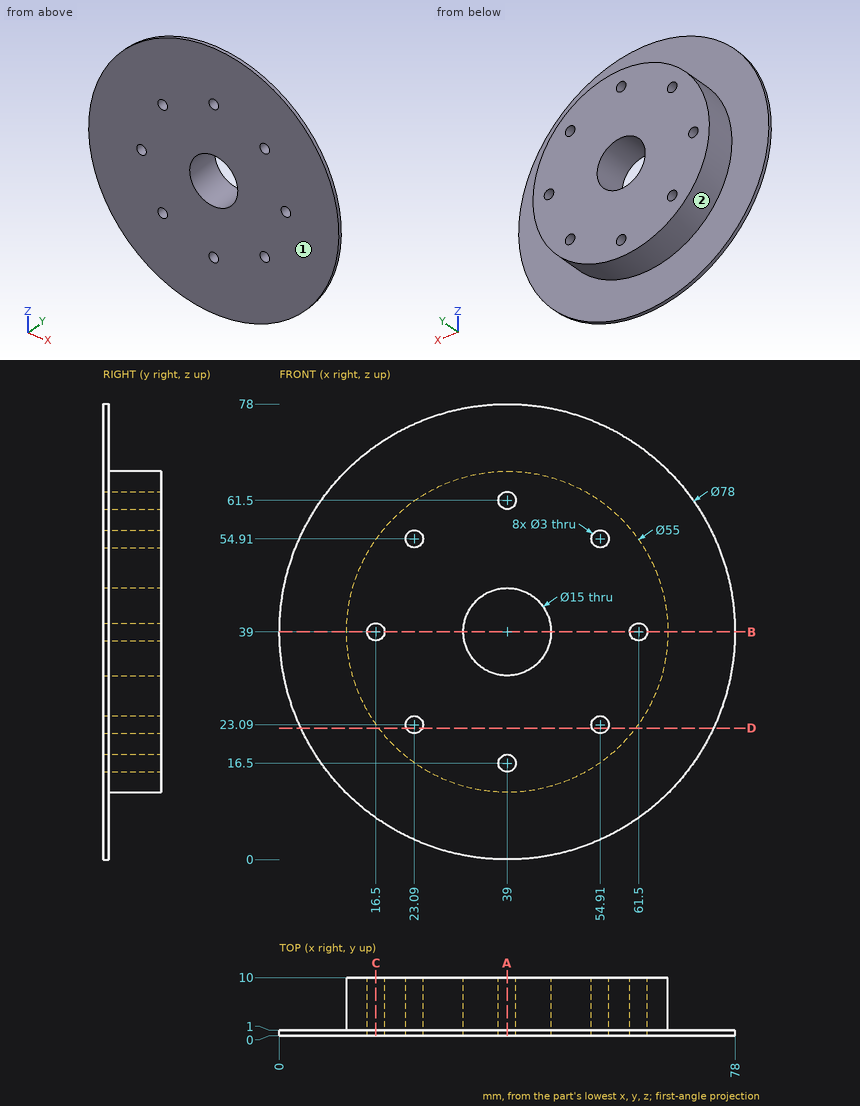
The figure shows three views and two pictorial views of one solid part (mm, origin at its lowest corner). Answer the questions. A direction names the side the tool comes from. Give positions to 0.01 mm unless a question says otherwise; leave off trailing zeros. Write each loop counter-clockwise with the first axis right and the second up, starting at its lowest first coordinate (ties: lowest second). Pieces come first, ordered by that corner, then holes. Notation, with made-up numbers: M 26.5,-11 L 71.5,-11 A24 cw 71.5,25 Z; hole C 8.5,45.25 d11. An arc over 180 degrees is marked long. One line per item, written item: value. Start each with the question number.
(1) Find section D-D (z = 22.5). Determine the outline of the cut face in (x, y).
(2) Find section C-C (x = 16.5). Determine the outline of the cut face in (y, z) (1 decimal), plus the area to 3 significant figures.
(3) Flat-ended cylindrical pins translate along their axes: pin 1 Ø3 at (y, z) = (6.5, 34.5) entering from +X; pin 2 Ø5 at (y, z) = (4, 62) entering from +X; pin 3 Ø5 at (y, z) = (4.5, 27) entering from -X. Find the tip coordinate at first contact, or state that the pin passes through.
(4) Find section B-B (z = 39). Determine the outline of the cut face in (x, y).
(5) Find section A-A (x = 39). Determine the outline of the cut face in (y, z).
(6) A tool of negligible diameter and unlimited length cuts with its end or side. For the marked faces 1 and 2, from which of +Z, -Z, +X, -X, +Y, -Y can it reach the whole face along a straight path? Write none if from no direction.
(7) Find the intervals of material crossed by line 1 (X direction, y = 2.5, z = 39); line 2 (X direction, y = 4.25, z = 54); line 3 (Z direction, x = 38.5, y = 1.75), in increasing order.
Results below:
1. outline: M 3.66,0 L 21.71,0 L 21.71,10 L 17,10 L 17,1 L 3.66,1 Z; M 24.47,0 L 53.53,0 L 53.53,10 L 24.47,10 Z; M 56.29,0 L 74.34,0 L 74.34,1 L 61,1 L 61,10 L 56.29,10 Z
2. outline: M 0,7.1 L 1,7.1 L 1,23.2 L 10,23.2 L 10,37.5 L 0,37.5 Z; M 0,40.5 L 10,40.5 L 10,54.8 L 1,54.8 L 1,70.9 L 0,70.9 Z
2. area: 318 mm^2
3. pin 1: stops at x = 66.34
3. pin 2: stops at x = 57.33
3. pin 3: stops at x = 13.19
4. outline: M 0,0 L 15,0 L 15,10 L 11.5,10 L 11.5,1 L 0,1 Z; M 18,0 L 31.5,0 L 31.5,10 L 18,10 Z; M 46.5,0 L 60,0 L 60,10 L 46.5,10 Z; M 63,0 L 78,0 L 78,1 L 66.5,1 L 66.5,10 L 63,10 Z
5. outline: M 0,0 L 1,0 L 1,11.5 L 10,11.5 L 10,15 L 0,15 Z; M 0,18 L 10,18 L 10,31.5 L 0,31.5 Z; M 0,46.5 L 10,46.5 L 10,60 L 0,60 Z; M 0,63 L 10,63 L 10,66.5 L 1,66.5 L 1,78 L 0,78 Z
6. face 1: +Z, -Z, +X, -X, -Y
6. face 2: +Y
7. line 1: x = 11.5 to 15, 18 to 31.5, 46.5 to 60, 63 to 66.5
7. line 2: x = 15.95 to 21.9, 24.28 to 53.72, 56.1 to 62.05
7. line 3: z = 11.5 to 15.09, 17.91 to 31.52, 46.48 to 60.09, 62.91 to 66.5
